from build123d import *

# Parameters (mm, degrees)
BOSS_EXTRUDE1_DEPTH = 20
CHAMFER1_SIZE       = 3
CUT_EXTRUDE1_START  = 1.014174
SKETCH2_R           = 4.2
CUT_EXTRUDE1_DEPTH  = 6


with BuildPart() as part:
    # Sketch1 → Boss-Extrude1 (new body)
    with BuildSketch(Plane.XY):
        with BuildLine():
            Line((-1.385825984, -1.366427285), (-2.461204781, -1.366427285))
            ThreePointArc((-2.461204781, -1.366427285), (-3.097600884, -1.630031182), (-3.361204781, -2.266427285))
            Line((-3.361204781, -2.266427285), (-3.361204781, -4.516427285))
            ThreePointArc((-3.361204781, -4.516427285), (-3.422936438, -4.608815239), (-3.531915459, -4.587137963))
            Line((-3.531915459, -4.587137963), (-6.124303615, -1.994749808))
            ThreePointArc((-6.124303615, -1.994749808), (-6.687912768, -1.151249101), (-6.885825984, -0.156272177))
            Line((-6.885825984, -0.156272177), (-6.885825984, 1.623417606))
            ThreePointArc((-6.885825984, 1.623417606), (-6.687912768, 2.61839453), (-6.124303615, 3.461895237))
            Line((-6.124303615, 3.461895237), (-3.531915459, 6.054283393))
            ThreePointArc((-3.531915459, 6.054283393), (-3.422936438, 6.075960668), (-3.361204781, 5.983572715))
            Line((-3.361204781, 5.983572715), (-3.361204781, 3.733572715))
            ThreePointArc((-3.361204781, 3.733572715), (-3.097600884, 3.097176612), (-2.461204781, 2.833572715))
            Line((-2.461204781, 2.833572715), (-1.385825984, 2.833572715))
            ThreePointArc((-1.385825984, 2.833572715), (-0.749429881, 3.097176612), (-0.485825984, 3.733572715))
            Line((-0.485825984, 3.733572715), (-0.485825984, 8.983572715))
            Line((-0.485825984, 8.983572715), (7.014174016, 8.983572715))
            Line((7.014174016, 8.983572715), (7.014174016, -7.516427285))
            Line((7.014174016, -7.516427285), (-0.485825984, -7.516427285))
            Line((-0.485825984, -7.516427285), (-0.485825984, -2.266427285))
            ThreePointArc((-0.485825984, -2.266427285), (-0.749429881, -1.630031182), (-1.385825984, -1.366427285))
        make_face()
    extrude(amount=BOSS_EXTRUDE1_DEPTH)

    # Chamfer1
    chamfer1_edges = [part.edges().sort_by_distance(p)[0] for p in [
        (7.014174016, 0.733572715, 20),
        (7.014174016, 0.733572715, 0),
        (7.014174016, 8.983572715, 10),
        (7.014174016, -7.516427285, 10),
    ]]
    chamfer(chamfer1_edges, length=CHAMFER1_SIZE)

    # Sketch2 (on Right Plane) → Cut-Extrude1 (cut)
    with BuildSketch(Plane(origin=(0, 0, 0), x_dir=(0, 0, -1), z_dir=(1, 0, 0)).offset(CUT_EXTRUDE1_START)):
        with Locations((-10, 0.733572715)):
            Circle(SKETCH2_R)
    extrude(amount=CUT_EXTRUDE1_DEPTH, mode=Mode.SUBTRACT)


solid = part.part
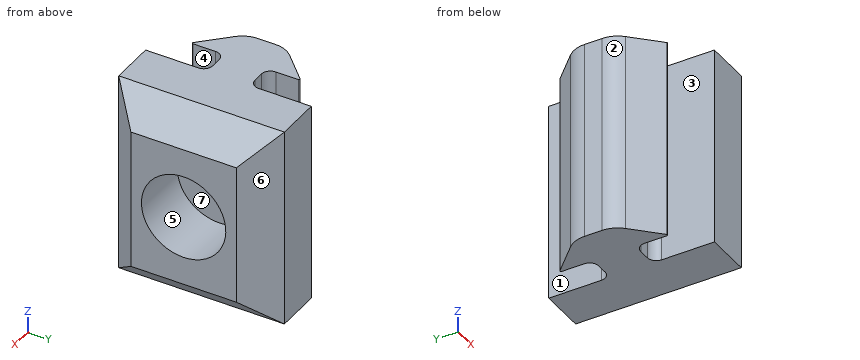
The model under review builds one solid part; all positions refer to its coordinate system, in mm. Face numbers are marked on the shaded views. A direction names the side the tool comes from. Give positions to 0.01 mm unless a question says otherwise; leave off trailing zeros. Loops run counter-clockwise (first coordinate to the right, second up) from the corner with the lowest first, then second, coordinate; pieces in that order, holes last. Notation, with made-up numbers: (-13, 85) -> (26, 85) arc R34 ccw to (26, 119) -> close; hole circle Ø8 at (19, -7.75). An arc over 180 degrees is marked (long way). Put each result on its own line as item: value. Start each with the question number.
1. Wall thickness on probe 1 along Y at (x, z) = (3.3, 10); probe 2 along X at (y, z) = (4.25, 1.5); probe 3 along X at (y, z) = (-2, 18.5): over which ranges is each line inside the solid? List them lowest first.
2. Mouldability with a two-part tool opening along Y and no side actions: class the marked faces 4, 5, 6 and 7 as released by +Y, released by -Y, zero draft, split by the parting line, or undercut.
3. We need section A-A on y = -4. State the section outline as (x, z) points, then the cut area to 3 significant figures.
4. We need section C-C on x = 2.25. State the section outline as (y, z) points.
5. We need section D-D on y = 2. State the section outline as (x, z) points.
6. For the marked faces 1, 2 and 3, list the 3-axis set-ups (+Z, -Z, +X, -X, +Y, -Y) from which the entire face can be reached by the end or side of a thin tool; tool diameter is ignored.
7. We need section B-B on z = 10. State the section outline as (x, y) points.
8. Clearance check with flat-ended pins moving along their axes: P1, Ø6.5, axis at y = 0.73, z = 10, coming from the +X side; P2, Ø4, axis at y = 5.5, z = 10, coming from the -X side; P3, Ø4, axis at y = 7, z = 7, coming from the -X side; P4, Ø1, axis at x = -2.5, y = -2.5, coming from the -Z side. State where each tip first meets the part, or that it passes through.
Determined:
1. probe 1: -7.52 to -3.47, 4.93 to 8.98
1. probe 2: -5.34 to -3.36, -0.49 to 5.51
1. probe 3: -6.12 to -3.32, -0.53 to 5.51
2. face 4: zero draft
2. face 5: undercut
2. face 6: released by +Y
2. face 7: undercut
3. outline: (-4.12, 0) -> (-3.36, 0) -> (-3.36, 20) -> (-4.12, 20) -> close; (-0.49, 0) -> (4.01, 0) -> (7.01, 3) -> (7.01, 17) -> (4.01, 20) -> (-0.49, 20) -> close
3. area: 156 mm^2
4. outline: (-7.52, 0) -> (8.98, 0) -> (8.98, 20) -> (-7.52, 20) -> close; hole circle Ø8.4 at (0.73, 10)
5. outline: (-6.86, 0) -> (4.01, 0) -> (7.01, 3) -> (7.01, 6) -> (1.01, 6) -> (1.01, 14) -> (7.01, 14) -> (7.01, 17) -> (4.01, 20) -> (-6.86, 20) -> close
6. face 1: +Z, -Z, +Y
6. face 2: +Z, -Z, -X, -Y
6. face 3: +Z, -Z, -Y
7. outline: (-6.89, -0.16) arc R2.6 ccw to (-6.12, -1.99) -> (-3.53, -4.59) arc R0.1 ccw to (-3.36, -4.52) -> (-3.36, -2.27) arc R0.9 cw to (-2.46, -1.37) -> (-1.39, -1.37) arc R0.9 cw to (-0.49, -2.27) -> (-0.49, -7.52) -> (4.01, -7.52) -> (7.01, -4.52) -> (7.01, -3.47) -> (1.01, -3.47) -> (1.01, 4.93) -> (7.01, 4.93) -> (7.01, 5.98) -> (4.01, 8.98) -> (-0.49, 8.98) -> (-0.49, 3.73) arc R0.9 cw to (-1.39, 2.83) -> (-2.46, 2.83) arc R0.9 cw to (-3.36, 3.73) -> (-3.36, 5.98) arc R0.1 ccw to (-3.53, 6.05) -> (-6.12, 3.46) arc R2.6 ccw to (-6.89, 1.62) -> close
8. P1: x = 1.01
8. P2: x = -6.09
8. P3: x = -4.59
8. P4: through
